CAD build for the part. Positions are in the model's coordinates, mm. A direction names the side the tool comes from. Round coordinates to 2 decimals unless told otherwise and drop trailing zeros. Loops run counter-clockwise (first coordinate to the right, second up) from the corner with the lowest first, then second, coordinate; pieces in that order, holes last. Notation, with made-up numbers: M 33,85 L 49,85 A15 ccw 49,96 Z; hole C -12.75,30 d9. An arc over 180 degrees is marked long. Put each result on its own line as item: value. Start each with the question number.
from build123d import *

# Parameters (mm, degrees)
F0_W      = 184
F0_H      = 100
F1_DEPTH  = 18
F2_W      = 86
F2_H      = 21.7137943208
F3_DEPTH  = 100.001
F5_DEPTH  = 92
F7_DEPTH  = 100
F8_R      = 86
F9_DEPTH  = 20
F10_START = -111
F10_DEPTH = 24
F12_W     = 146
F12_H     = 103
F13_DEPTH = 92
F15_DEPTH = 103
F16_W     = 126
F16_H     = 83
F17_DEPTH = 59.2595889125


with BuildPart() as f1:
    # F0 (on Top) → F1 (new body)
    with BuildSketch(Plane.XY):
        with Locations((0, 65)):
            Rectangle(F0_W, F0_H)
    extrude(amount=F1_DEPTH)

    # F2 (on face) → F3 (cut, through all)
    with BuildSketch(Plane.XZ.offset(-15)):
        with Locations((0, -5.8568971604)):
            Rectangle(F2_W, F2_H)
    extrude(amount=-F3_DEPTH, mode=Mode.SUBTRACT)

    # F4 (on face) → F5 (join)
    with BuildSketch(Plane.XY.offset(18)):
        Polygon((-63, 57), (-63, 15), (-49, 15), (-49, 57), (0, 57), (49, 57), (49, 15), (63, 15), (63, 57), (73, 57), (73, 69), (63, 69), (63, 115), (49, 115), (49, 69), (0, 69), (-49, 69), (-49, 115), (-63, 115), (-63, 69), (-73, 69), (-73, 57), align=None)
    extrude(amount=F5_DEPTH)

    # F6 (on face) → F7 (join)
    with BuildSketch(Plane.XZ.offset(-15)):
        with BuildLine():
            Line((-73, 120), (-73, 84.9001424504))
            ThreePointArc((-73, 84.9001424504), (0, 39), (73, 84.9001424504))
            Line((73, 84.9001424504), (73, 120))
            Line((73, 120), (-73, 120))
        make_face()
    extrude(amount=-F7_DEPTH)

    # F8 (on Front) → F9 (join)
    with BuildSketch(Plane.XZ):
        with Locations((0, 120)):
            Circle(F8_R)
    extrude(amount=-F9_DEPTH)

    # F8 (on Front) → F10 (join)
    with BuildSketch(Plane.XZ.offset(F10_START)):
        with Locations((0, 120)):
            Circle(F8_R)
    extrude(amount=-F10_DEPTH)

    # F12 (on offset) → F13 (join, through all)
    with BuildSketch(Plane.XY.offset(212)):
        with Locations((0, 61.5)):
            Rectangle(F12_W, F12_H)
    extrude(amount=-F13_DEPTH)

    # F14 (on face) → F15 (cut)
    with BuildSketch(Plane.XZ):
        with BuildLine():
            Line((-63, 152.7414110875), (-63, 87.2585889125))
            ThreePointArc((-63, 87.2585889125), (0, 49), (63, 87.2585889125))
            Line((63, 87.2585889125), (63, 152.7414110875))
            ThreePointArc((63, 152.7414110875), (0, 191), (-63, 152.7414110875))
        make_face()
    extrude(amount=-F15_DEPTH, mode=Mode.SUBTRACT)

    # F16 (on face) → F17 (cut, through all)
    with BuildSketch(Plane.XY.offset(212)):
        with Locations((0, 61.5)):
            Rectangle(F16_W, F16_H)
    extrude(amount=-F17_DEPTH, mode=Mode.SUBTRACT)


solid = f1.part
(1) Tool access for faces 4 (the cylindrical face through (68.388, 38.241, 76.594)), 5 (the flat face through (-1, 10, 210)), 6 (the flat face through (-73, 61, 138)), 7 (the flat face through (-1, 92, 18)), 8 (the flat face through (-1, 113, 210)): list every direction of +Z, -Z, +X, -X, +Y, -Y with a clear straight run to the whole face (end or side of a thin tool).
(2) Cut at D-D on x = -80. List the corners of the cut face in (y, z), and give its area (3 significant figures).
(3) Cut at A-A on x = 0. List the corners of the cut face in (y, z), and give its area (3 significant figures).
(4) Flat gauge pins, fed straight in: pin 1 Ø3 at (y, z) = (116, 84.5) entering from -X; pin 2 Ø8 at (y, z) = (38.5, 155.5) entering from +X; pin 3 Ø4 at (x, y) = (37, 89) entering from -Z. Where does each tip first touch, or does it go through?
(5) Drill centre lines: line 1 along X through (y, z) = (24.5, 141); line 2 along Y through (x, z) = (-84, 123.5); line 3 along Y through (x, z) = (-44, 94). Where is each one in solid material? Low to high.
(6) Mould opens along X. For faces 1 (the flat face through (79, 111, 114)), 2 (the flat face through (0, 20, 38)), 3 (the flat face through (73, 61, 138)) say: +X half, -X half, draft (parallel to the pull), parting line (faces both ways), or undercut.
(7) Cut at B-B on y = 32. List the corners of the cut face in (x, z).
(8) Cut at C-C on z = 120. List the corners of the cut face in (x, y), and give its area (3 significant figures).
Taken from the geometry:
1. face 4: +X
1. face 5: +Z, -Y
1. face 6: +Z, -X
1. face 7: +Y
1. face 8: +Z, +Y
2. outline: M 0,88.44 L 20,88.44 L 20,151.56 L 0,151.56 Z; M 15,0 L 115,0 L 115,18 L 15,18 Z; M 111,88.44 L 135,88.44 L 135,151.56 L 111,151.56 Z
2. area: 4,580 mm2
3. outline: M 0,34 L 20,34 L 20,39 L 57,39 L 57,18 L 15,18 L 15,5 L 115,5 L 115,18 L 69,18 L 69,39 L 111,39 L 111,34 L 135,34 L 135,206 L 113,206 L 113,212 L 103,212 L 103,49 L 0,49 Z; M 0,191 L 20,191 L 20,212 L 10,212 L 10,206 L 0,206 Z
3. area: 8,570 mm2
4. pin 1: x = -78.99
4. pin 2: x = 73
4. pin 3: z = 5
5. line 1: -73 to -63, 63 to 73
5. line 2: 0 to 20, 111 to 135
5. line 3: 103 to 135
6. face 1: draft
6. face 2: undercut
6. face 3: +X half
7. outline: M -92,0 L -43,0 L -43,5 L 43,5 L 43,0 L 92,0 L 92,18 L 63,18 L 63,69.09 A81 ccw 73,84.9 L 73,212 L 63,212 L 63,87.26 A71 cw -63,87.26 L -63,212 L -73,212 L -73,84.9 A81 ccw -63,69.09 L -63,18 L -92,18 Z; hole M -49,18 L 49,18 L 49,55.5 A81 cw -49,55.5 Z
8. outline: M -86,0 L -63,0 L -63,103 L 63,103 L 63,0 L 86,0 L 86,20 L 73,20 L 73,111 L 86,111 L 86,135 L -86,135 L -86,111 L -73,111 L -73,20 L -86,20 Z
8. area: 7,880 mm2
